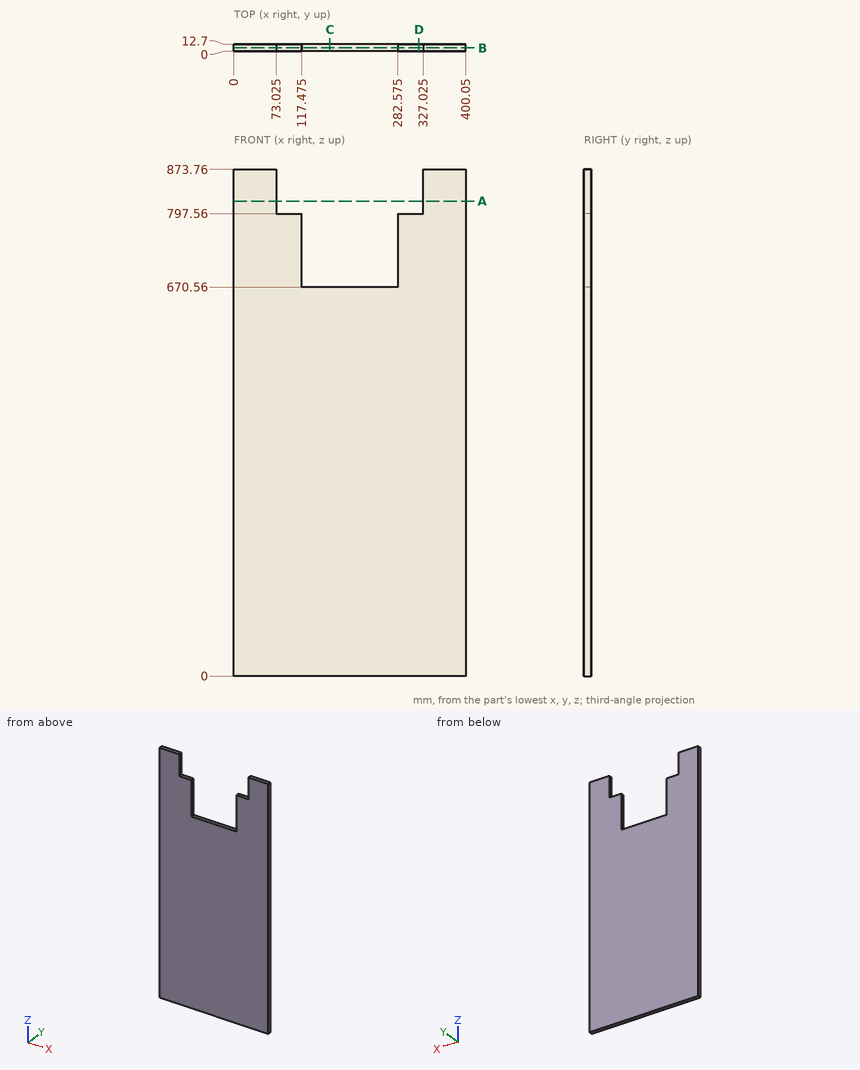
The drawing under review shows one solid part. Ordinate dimensions are in mm from its lowest x, y, z. Coordinates: 2 decimals unless noted, no trailing zeros. Write each loop counter-clockwise with the first axis right and the second up, starting at its lowest first coordinate (ties: lowest second). Pieces come first, ordered by that corner, then holes. Notation, with made-up numbers: (44.25, 43.5) - (54.25, 43.5) arc R6 cw to (54.25, 51.5) - close; hole circle Ø10 at (51, -31.5). An arc over 180 degrees is marked (long way). Put each result on its own line as item: value.
1. Add section C-C, the plane x = 165.5. Give the boundary of the cut face in (y, z), then the cut area to 3 significant figures.
Values found:
outline: (0, 0) - (12.7, 0) - (12.7, 670.56) - (0, 670.56) - close
area: 8,520 mm²
2. Add section A-A, the plane z = 819. Give the boundary of the cut face in (x, y) (3 decimals), then the cut area to 3 significant figures.
Values found:
outline: (0, 0) - (73.025, 0) - (73.025, 12.7) - (0, 12.7) - close; (327.025, 0) - (400.05, 0) - (400.05, 12.7) - (327.025, 12.7) - close
area: 1,850 mm²
3. Wall thickness on probe 1 along X at (y, z) = (9, 676.5) (3 decimals); probe 2 along Z at (x, y) = (205, 2); probe 3 along Z at (x, y) = (90, 8): over which ranges is each line inside the solid? List them lowest first.
Values found:
probe 1: 0 to 117.475, 282.575 to 400.05
probe 2: 0 to 670.56
probe 3: 0 to 797.56
4. Add section B-B, the plane y = 6. Give the boundary of the cut face in (x, z) (3 decimals), then the cut area to 3 significant figures.
Values found:
outline: (0, 0) - (400.05, 0) - (400.05, 873.76) - (327.025, 873.76) - (327.025, 797.56) - (282.575, 797.56) - (282.575, 670.56) - (117.475, 670.56) - (117.475, 797.56) - (73.025, 797.56) - (73.025, 873.76) - (0, 873.76) - close
area: 309,000 mm²
5. For pin 1 (4 mm diameter, centred on x = 279.5, y = 3, fed in from -Z); pin 2 (4 mm diameter, centred on x = 303.5, y = 4.5, fed in from +Z); pin 3 (6.5 mm diameter, centred on x = 202, y = 9, fed in from +Z), all flat-tipped, find the tip position at first contact; note any pin that passes through.
Values found:
pin 1: z = 0
pin 2: z = 797.56
pin 3: z = 670.56
6. Add section D-D, the plane x = 319. Give the boundary of the cut face in (y, z).
Values found:
outline: (0, 0) - (12.7, 0) - (12.7, 797.56) - (0, 797.56) - close
